from build123d import *

# Parameters (mm, degrees)
SKETCH1_W           = 285
SKETCH1_H           = 17.2
SKETCH1_R           = 4.6
SKETCH1_H_2         = 3.16
SKETCH1_R_2         = 2.55
BOSS_EXTRUDE1_DEPTH = 5
BOSS_EXTRUDE2_START = 5
SKETCH1_3_W         = 285
SKETCH1_3_H         = 3.16
BOSS_EXTRUDE2_DEPTH = 16
CUT_EXTRUDE1_START  = 2.8
SKETCH1_5_R         = 4.6
SKETCH1_5_R_2       = 2.55
CUT_EXTRUDE1_DEPTH  = 2.2


with BuildPart() as part:
    # Sketch1 → Boss-Extrude1 (new body)
    # profile 1 of 4: a face of its own
    with BuildSketch(Plane(origin=(0, 0, 0), x_dir=(1, 0, 0), z_dir=(0, 1, 0))):
        with Locations((0, -1.58)):
            Rectangle(SKETCH1_W, SKETCH1_H)
        with Locations((-132.5, 0)):
            Circle(SKETCH1_R, mode=Mode.SUBTRACT)
        with Locations((132.5, 0)):
            Circle(SKETCH1_R, mode=Mode.SUBTRACT)
    # profile 2 of 4: a face of its own
    with BuildSketch(Plane(origin=(0, 0, 0), x_dir=(1, 0, 0), z_dir=(0, 1, 0))):
        with Locations((0, 8.6)):
            Rectangle(SKETCH1_W, SKETCH1_H_2)
    # profile 3 of 4: a face of its own
    with BuildSketch(Plane(origin=(0, 0, 0), x_dir=(1, 0, 0), z_dir=(0, 1, 0))):
        with Locations((-132.5, 0)):
            Circle(SKETCH1_R)
        with Locations(Location((-132.5, 0, 0), (0, 0, 270))):
            Circle(SKETCH1_R_2, mode=Mode.SUBTRACT)
    # profile 4 of 4: a face of its own
    with BuildSketch(Plane(origin=(0, 0, 0), x_dir=(1, 0, 0), z_dir=(0, 1, 0))):
        with Locations((132.5, 0)):
            Circle(SKETCH1_R)
        with Locations(Location((132.5, 0, 0), (0, 0, 270))):
            Circle(SKETCH1_R_2, mode=Mode.SUBTRACT)
    extrude(amount=BOSS_EXTRUDE1_DEPTH)

    # Sketch1<3> → Boss-Extrude2 (add)
    with BuildSketch(Plane(origin=(0, 0, 0), x_dir=(1, 0, 0), z_dir=(0, 1, 0)).offset(BOSS_EXTRUDE2_START)):
        with Locations((0, 8.6)):
            Rectangle(SKETCH1_3_W, SKETCH1_3_H)
    extrude(amount=BOSS_EXTRUDE2_DEPTH)

    # Sketch1<5> → Cut-Extrude1 (cut)
    # profile 1 of 2: a face of its own
    with BuildSketch(Plane(origin=(0, 0, 0), x_dir=(1, 0, 0), z_dir=(0, 1, 0)).offset(CUT_EXTRUDE1_START)):
        with Locations(Location((-132.5, 0, 0), (0, 0, 270))):
            Circle(SKETCH1_5_R)
        with Locations(Location((-132.5, 0, 0), (0, 0, 270))):
            Circle(SKETCH1_5_R_2, mode=Mode.SUBTRACT)
    # profile 2 of 2: a face of its own
    with BuildSketch(Plane(origin=(0, 0, 0), x_dir=(1, 0, 0), z_dir=(0, 1, 0)).offset(CUT_EXTRUDE1_START)):
        with Locations(Location((132.5, 0, 0), (0, 0, 270))):
            Circle(SKETCH1_5_R)
        with Locations(Location((132.5, 0, 0), (0, 0, 270))):
            Circle(SKETCH1_5_R_2, mode=Mode.SUBTRACT)
    extrude(amount=CUT_EXTRUDE1_DEPTH, mode=Mode.SUBTRACT)


solid = part.part
CAD build for the part. Positions are in the model's coordinates, mm. A direction names the side the tool comes from. Give positions to 0.01 mm unless a question says otherwise; leave off trailing zeros. Order: outer loops, then holes, each group sorted by start corner. A loop starts at its lowest first (then second) coordinate and runs counter-clockwise, first axis right, second up. Notation, with made-up numbers: (35.5, 73) - (93.5, 73) arc R20 cw to (93.5, 103) - close; hole circle Ø11 at (0, 63). An arc over 180 degrees is marked (long way). Answer in a Markdown table with one row per item.
1. Saw through at C-C, the plane x = -77.5. Give the cut face in (y, z).
Data:
| item | result |
|---|---|
| outline | (0, -10.18) - (21, -10.18) - (21, -7.02) - (5, -7.02) - (5, 10.18) - (0, 10.18) - close |
2. Saw through at A-A, the plane z = 0. Give the cut face in (x, y).
Data:
| item | result |
|---|---|
| outline | (-142.5, 0) - (-135.05, 0) - (-135.05, 2.8) - (-137.1, 2.8) - (-137.1, 5) - (-142.5, 5) - close; (-129.95, 0) - (129.95, 0) - (129.95, 2.8) - (127.9, 2.8) - (127.9, 5) - (-127.9, 5) - (-127.9, 2.8) - (-129.95, 2.8) - close; (135.05, 0) - (142.5, 0) - (142.5, 5) - (137.1, 5) - (137.1, 2.8) - (135.05, 2.8) - close |
3. Pull direction X, two halves, no side cores. Call faces 1 (the cylindrical face through (135.03, 1.38, -0.33)), 2 (the flat face through (-142.5, 4, -2)), 3 (the flat face through (-2, 13, -7.02)): pulls with the +X half, pulls with the -X half, needs draft (parallel to the pull), parting line crosses it, or undercut.
Data:
| item | result |
|---|---|
| face 1 | undercut |
| face 2 | pulls with the -X half |
| face 3 | needs draft |
4. Saw through at B-B, the plane x = -132.5. Give the cut face in (y, z), plus the area to 3 significant figures.
Data:
| item | result |
|---|---|
| outline | (0, -10.18) - (21, -10.18) - (21, -7.02) - (5, -7.02) - (5, -4.6) - (2.8, -4.6) - (2.8, -2.55) - (0, -2.55) - close; (0, 2.55) - (2.8, 2.55) - (2.8, 4.6) - (5, 4.6) - (5, 10.18) - (0, 10.18) - close |
| area | 118 mm² |
5. Saw through at D-D, the plane y = 10.75. Give the cut face in (x, z), plus the area to 3 significant figures.
Data:
| item | result |
|---|---|
| outline | (-142.5, -10.18) - (142.5, -10.18) - (142.5, -7.02) - (-142.5, -7.02) - close |
| area | 901 mm² |
6. Flat gauge pins, fed straight in: pin 1 (5 mm diameter, centred on x = 53.5, z = -0.5, fed in from +Y); pin 2 (3 mm diameter, centred on x = 131, z = -2.5, fed in from +Y); pin 3 (4 mm diameter, centred on x = -132.5, z = 0, fed in from +Y); pin 4 (5 mm diameter, centred on x = -45.5, y = 9.5, fed in from +Z). Where does each tip first touch, or does it go through?
Data:
| item | result |
|---|---|
| pin 1 | stops at y = 5 |
| pin 2 | stops at y = 2.8 |
| pin 3 | passes through |
| pin 4 | stops at z = -7.02 |
7. Tool access for faces 4 (the cylindrical face through (-136.99, 3.88, -1)), 5 (the flat face through (-2, 5, 1)), 6 (the flat face through (142.5, 4, -2)): list every direction of +Z, -Z, +X, -X, +Y, -Y with a clear straight run to the whole face (end or side of a thin tool).
Data:
| item | result |
|---|---|
| face 4 | +Y |
| face 5 | +Z, +X, -X, +Y |
| face 6 | +Z, -Z, +X, +Y, -Y |
8. Probe probe 1 along X at (y, z) = (1.2, 0); probe 2 along X at (y, z) = (3.5, 0); probe 3 along Z at (x, y) = (-132.5, 0.6). List the from-to ranges inside material, lowest first. Write a range as [from, to].
Data:
| item | result |
|---|---|
| probe 1 | x = [-142.5, -135.05], [-129.95, 129.95], [135.05, 142.5] |
| probe 2 | x = [-142.5, -137.1], [-127.9, 127.9], [137.1, 142.5] |
| probe 3 | z = [-10.18, -2.55], [2.55, 10.18] |
